from build123d import *

# Parameters (mm, degrees)
BOSS_EXTRUDE1_DEPTH = 5.75
CIRPATTERN1_COUNT   = 20
SKETCH2_R           = 11.945
BOSS_EXTRUDE2_DEPTH = 1.5
SKETCH3_R           = 3.2
CUT_EXTRUDE1_DEPTH  = 14.5


with BuildPart() as part:
    # Sketch1 → Boss-Extrude1 (new, symmetric)
    with BuildSketch(Plane(origin=(0, 0, 0), x_dir=(0, 0, -1), z_dir=(1, 0, 0))):
        with BuildLine():
            Line((0, 13.285), (0, 0))
            Line((0, 0), (4.10529077, 12.634785819))
            ThreePointArc((4.10529077, 12.634785819), (3.221971668, 13.384600745), (3.120582785, 14.538808418))
            ThreePointArc((3.120582785, 14.538808418), (3.07819699, 14.888914891), (2.788180956, 15.089568316))
            ThreePointArc((2.788180956, 15.089568316), (2.400486866, 15.156077586), (2.011215381, 15.212627574))
            ThreePointArc((2.011215381, 15.212627574), (1.673388423, 15.111414709), (1.524888287, 14.791541599))
            ThreePointArc((1.524888287, 14.791541599), (1.071791943, 13.725155757), (0, 13.285))
        make_face()
    boss_extrude1 = extrude(amount=BOSS_EXTRUDE1_DEPTH, both=True)

    # CirPattern1: Boss-Extrude1 ×20 about axis
    cirpattern1_axis = Axis((0, 0, 0), (1, 0, 0))
    for i in range(1, CIRPATTERN1_COUNT):
        add(boss_extrude1.rotate(cirpattern1_axis, i * 360 / CIRPATTERN1_COUNT))

    # Sketch2 → Boss-Extrude2 (add)
    with BuildSketch(Plane(origin=(5.75, 0, 0), x_dir=(0, 0, -1), z_dir=(1, 0, 0))):
        Circle(SKETCH2_R)
    boss_extrude2 = extrude(amount=BOSS_EXTRUDE2_DEPTH)

    # Mirror1: Boss-Extrude2 across plane
    add(boss_extrude2.mirror(Plane(origin=(0, 0, 0), x_dir=(0, 0, 1), z_dir=(1, 0, 0))))

    # Sketch3 → Cut-Extrude1 (cut)
    with BuildSketch(Plane(origin=(7.25, 0, 0), x_dir=(0, 0, -1), z_dir=(1, 0, 0))):
        Circle(SKETCH3_R)
    extrude(amount=-CUT_EXTRUDE1_DEPTH, mode=Mode.SUBTRACT)


solid = part.part
Build history of the part. All positions in model axes, mm. A direction names the side the tool comes from. Round coordinates to 2 decimals unless told otherwise and drop trailing zeros. Write each loop counter-clockwise with the first axis right and the second up, starting at its lowest first coordinate (ties: lowest second). Pieces come first, ordered by that corner, then holes. Notation, with made-up numbers: M -13.5,-19 L 18.5,-19 A20 ccw 18.5,2 Z; hole C -11.75,-14 d4. An arc over 180 degrees is marked long. Answer in a Markdown table with one row per item.
1. Probe L1, parallel to Y at x = -6.5, z = 0 (3 decimals); L2, parallel to Y at x = -1.75, z = -11.5; L3, parallel to X at y = 11, z = 10.5. List the from-to ranges inside material, lowest first. Write a range as [from, to].
Geometry check:
| item | result |
|---|---|
| L1 | [-11.945, -3.2], [3.2, 11.945] |
| L2 | [-7.26, 7.26] |
| L3 | [-5.75, 5.75] |
2. Saw through at A-A (x = 6.25). List the corners of the cut face in (y, z) (3 decimals), and give its area (3 significant figures).
Geometry check:
| item | result |
|---|---|
| outline | C 0,0 d23.89; hole C 0,0 d6.4 |
| area | 416 mm2 |
3. Mould opens along Z. For faces 4 (the face through (6.49, -7.27, 9.48)), 5 (the face through (0.101, -1.947, 2.539)), 6 (the face through (7.25, -2.5, -2.5)) say: +Z half, -Z half, draft (parallel to the pull), parting line (faces both ways), or undercut.
Geometry check:
| item | result |
|---|---|
| face 4 | parting line |
| face 5 | undercut |
| face 6 | draft |
4. Which spindle directions (+Z, -Z, +X, -X, +Y, -Y) get a long thin tool onto all of the face, cutting with end or side? Do faces 1 (the face through (-7.25, -2.5, -2.5)), 2 (the face through (-5.75, 10.4, 6.2)), 3 (the face through (5.75, 10.4, 6.2)). Say none if no direction does.
Geometry check:
| item | result |
|---|---|
| face 1 | +Z, -Z, -X, +Y, -Y |
| face 2 | -X |
| face 3 | +X |
5. Flat gauge pins, fed straight in: P1, Ø4, axis at x = -4.5, y = 7.5, coming from the +Z side; P2, Ø1.5, axis at x = -2.5, y = 10, coming from the +Z side; P3, Ø1, axis at x = -5.5, z = -4.5, coming from the +Y side. Where does each tip first touch, or does it go through?
Geometry check:
| item | result |
|---|---|
| P1 | z = 13.89 |
| P2 | z = 11.24 |
| P3 | y = 12.67 |
